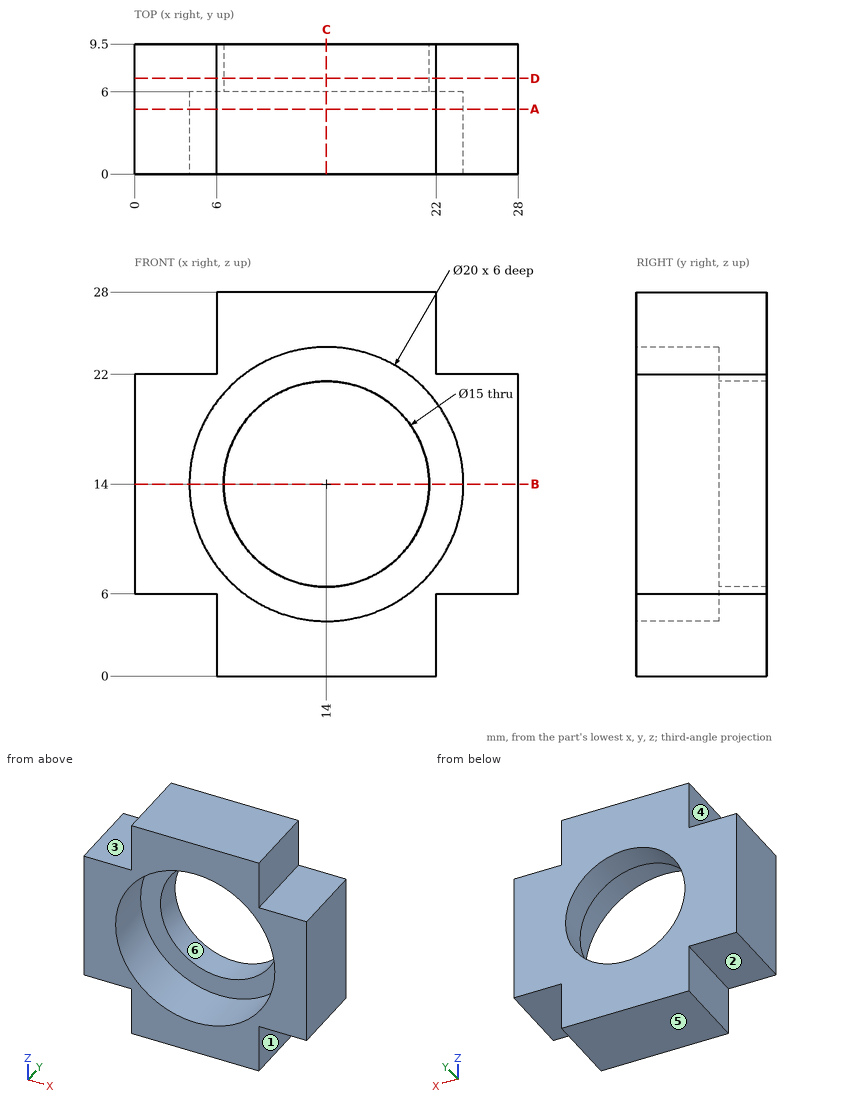
Can you work these out from the drawing? Everything is in mm from the part's minimum corner. A direction names the side the tool comes from. Round coordinates to 2 decimals unless told otherwise and drop trailing zeros. Loops run counter-clockwise (first coordinate to the right, second up) from the corner with the lowest first, then second, coordinate; pieces in that order, holes last. Notation, with made-up numbers: (9, 65.25) - (15, 65.25) arc R28 ccw to (15, 100.25) - close; hole circle Ø8 at (7.5, 22). An arc over 180 degrees is marked (long way). Answer in a Markdown table with one row per item. Add a question column.
Q1. I want a section at B-B on z = 14. List the corners of the cut face in (x, y) for me, and give its area (3 significant figures).
Q2. I want a section at D-D on y = 7. List the corners of the cut face in (x, z) for me, and give its area (3 significant figures).
Q3. I need wall thicknesses on L1, parallel to Z at x = 8, y = 0.5; L2, parallel to X at y = 3.75, z = 24.25; L3, parallel to X at y = 7.55, z = 14. Which ranges of each line are inside material? Lowest first, please.
Q4. We'd pull the mould along X, two halves only. Please class the marked faces 4, 5 and 6: pulls with the +X half, pulls with the -X half, needs draft (parallel to the pull), parting line crosses it, or undercut.
Q5. For pin 1 Ø10 at (x, z) = (15.5, 18.5) entering from -Y; pin 2 Ø2 at (x, y) = (18, 2.5) entering from -Z; pin 3 Ø5 at (x, y) = (2, 2.5) entering from +Z; pin 4 Ø3 at (y, z) = (2.5, 4) entering from +X, each with a flat end and sliding along its axis, tell me the tip position at first contact or that it passes through.
Q6. I want a section at C-C on x = 14. List the corners of the cut face in (y, z) for me, and give its area (3 significant figures).
Q7. Which directions (+Z, -Z, +X, -X, +Y, -Y) give clear straight access to the entire face, cutting with the end or side of a thin tool? Please do the marked faces 1, 2 and 3.
Q8. I want a section at A-A on y = 4.75. List the corners of the cut face in (x, z) for me, and give its area (3 significant figures).
A:
| question | item | result |
|---|---|---|
| 1 | outline | (0, 0) - (4, 0) - (4, 6) - (6.5, 6) - (6.5, 9.5) - (0, 9.5) - close; (21.5, 6) - (24, 6) - (24, 0) - (28, 0) - (28, 9.5) - (21.5, 9.5) - close |
| 1 | area | 93.5 mm^2 |
| 2 | outline | (0, 6) - (6, 6) - (6, 0) - (22, 0) - (22, 6) - (28, 6) - (28, 22) - (22, 22) - (22, 28) - (6, 28) - (6, 22) - (0, 22) - close; hole circle Ø15 at (14, 14) |
| 2 | area | 463 mm^2 |
| 3 | L1 | 0 to 6, 22 to 28 |
| 3 | L2 | 6 to 22 |
| 3 | L3 | 0 to 6.5, 21.5 to 28 |
| 4 | face 4 | pulls with the -X half |
| 4 | face 5 | needs draft |
| 4 | face 6 | undercut |
| 5 | pin 1 | y = 6 |
| 5 | pin 2 | z = 0 |
| 5 | pin 3 | z = 22 |
| 5 | pin 4 | x = 22 |
| 6 | outline | (0, 0) - (9.5, 0) - (9.5, 6.5) - (6, 6.5) - (6, 4) - (0, 4) - close; (0, 24) - (6, 24) - (6, 21.5) - (9.5, 21.5) - (9.5, 28) - (0, 28) - close |
| 6 | area | 93.5 mm^2 |
| 7 | face 1 | -Z, +X, +Y, -Y |
| 7 | face 2 | -Z, -X, +Y, -Y |
| 7 | face 3 | +Z, -X, +Y, -Y |
| 8 | outline | (0, 6) - (6, 6) - (6, 0) - (22, 0) - (22, 6) - (28, 6) - (28, 22) - (22, 22) - (22, 28) - (6, 28) - (6, 22) - (0, 22) - close; hole circle Ø20 at (14, 14) |
| 8 | area | 326 mm^2 |
